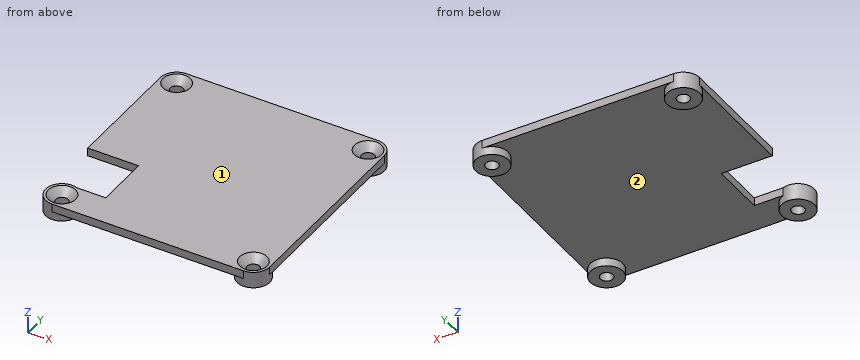
Autodesk Fusion 360 part; units mm, degrees
sketch "Sketch1" plane through (0, 0, 0) normal (0, 0, 1) x (1, 0, 0)
  line L0 (0, 0) -> (55, 0)
  line L1 (55, 0) -> (55, 55)
  line L2 (55, 55) -> (0, 55)
  line L3 (0, 55) -> (0, 0)
  circle A0 centre (4, 51) radius 4
  circle A1 centre (51, 51) radius 4
  circle A2 centre (4, 4) radius 4
  circle A3 centre (51, 4) radius 4
  circle A4 centre (4, 51) radius 1.55
  circle A5 centre (51, 51) radius 1.55
  circle A6 centre (4, 4) radius 1.55
  circle A7 centre (51, 4) radius 1.55
  line L4 (0, 21.25) -> (12.5, 21.25)
  line L5 (12.5, 21.25) -> (12.5, 7.75)
  line L6 (12.5, 7.75) -> (0, 7.75)
  line L7 (0, 7.75) -> (0, 21.25)
  dimension "d1" = 55
  dimension "d2" = 55
  dimension "d3" = 8
  dimension "d4" = 8
  dimension "d5" = 8
  dimension "d6" = 8
  dimension "d7" = 4
  dimension "d8" = 4
  dimension "d9" = 4
  dimension "d10" = 4
  dimension "d11" = 4
  dimension "d12" = 4
  dimension "d13" = 4
  dimension "d14" = 4
  dimension "d15" = 3.1
  dimension "d16" = 3.1
  dimension "d17" = 3.1
  dimension "d18" = 3.1
  dimension "d24" = 12.5
  dimension "d25" = 13.5
  dimension "d26" = 7.75
extrude "Extrude3" add sketch "Sketch1" against normal blind 2 contours L0 L1 L2 L3 A0 A1 A2 A3 L4 L5 L6
extrude "Extrude4" add sketch "Sketch1" against normal blind 4 contours A2 L6 | A3 | A2 L6 | A1 | A0
chamfer "Chamfer2" distance 1.8 angle 45 4 edges at (2.5549, 51.5605, 0) (49.5549, 51.5605, 0) (49.5549, 4.5605, 0) (2.5549, 4.5605, 0)
CAD build for the part. Positions are in the model's coordinates, mm. Face numbers are marked on the shaded views. Coordinates: 2 decimals unless noted, no trailing zeros. Order: outer loops, then holes, each group sorted by start corner. A loop starts at its lowest first (then second) coordinate and runs counter-clockwise, first axis right, second up. Notation, with made-up numbers: (20.25, -2) - (28.25, -2) arc R31 cw to (28.25, 29) - close; hole circle Ø6 at (43, 34). An arc over 180 degrees is marked (long way). Use a Markdown table: item, result. Add a question column.
(1) Saw through at A-A (z = -3.05). Give the cut face in (x, y).
(2) Drill centre lines: line 1 along Y through (x, z) = (51, -2.7); line 2 along Y through (x, z) = (49.5, -1.6); line 3 along Z through (x, y) = (21.5, 26). Where is each one in solid material? Low to high. Write a range as [from, to].
(3) Pull direction X, two halves, no side cores. Call the marked faces 1 and 2: +X half, -X half, draft (parallel to the pull), parting line (faces both ways), or undercut.
(4) Saw through at B-B (x = 42.5). Give the cut face in (y, z).
(5) Flat gauge pins, fed straight in: pin 1 (5 mm diameter, centred on x = 7.5, y = 27, fed in from -Z); pin 2 (0.6 mm diameter, centred on y = 15, z = -0.5, fed in from -X); pin 3 (4 mm diameter, centred on x = 51, y = 4, fed in from +Z). Where does each tip first touch, or does it go through?
(6) Saw through at C-C (y = 19.5). Give the cut face in (x, z).
Solved:
| question | item | result |
|---|---|---|
| 1 | outline | circle Ø8 at (4, 4); circle Ø8 at (4, 51); circle Ø8 at (51, 4); circle Ø8 at (51, 51); hole circle Ø3.1 at (4, 4); hole circle Ø3.1 at (4, 51); hole circle Ø3.1 at (51, 4); hole circle Ø3.1 at (51, 51) |
| 2 | line 1 | y = [0, 2.45], [5.55, 8], [47, 49.45], [52.55, 55] |
| 2 | line 2 | y = [0, 3.1], [4.9, 50.1], [51.9, 55] |
| 2 | line 3 | z = [-2, 0] |
| 3 | face 1 | draft |
| 3 | face 2 | undercut |
| 4 | outline | (0, -2) - (55, -2) - (55, 0) - (0, 0) - close |
| 5 | pin 1 | stops at z = -2 |
| 5 | pin 2 | stops at x = 12.5 |
| 5 | pin 3 | stops at z = -1.35 |
| 6 | outline | (12.5, -2) - (55, -2) - (55, 0) - (12.5, 0) - close |
